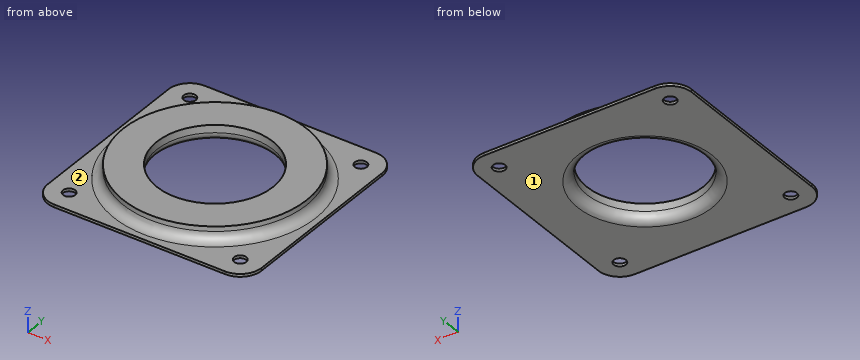
Autodesk Inventor part; units mm, degrees
ref_plane "YZ Plane" through (0, 0, 0) normal (1, 0, 0) x (0, 1, 0)
ref_plane "XZ Plane" through (0, 0, 0) normal (0, 1, 0) x (-1, 0, 0)
ref_plane "XY Plane" through (0, 0, 0) normal (0, 0, 1) x (1, 0, 0)
sketch "Skizze1" plane through (0, 0, 0) normal (0, 0, 1) x (1, 0, 0)
  line L0 (-35, 35) -> (35, 35)
  line L1 (35, 35) -> (35, -35)
  line L2 (35, -35) -> (-35, -35)
  line L3 (-35, -35) -> (-35, 35)
  circle A0 centre (0, 0) radius 35
  circle A1 centre (0, 0) radius 19
  dimension "d0" = 70
  dimension "d1" = 38
extrude "Extrusion1" add sketch "Skizze1" along normal blind 0.9
fillet "Rundung1" radius 7 4 edges at (-35, -35, 0.45) (35, -35, 0.45) (-35, 35, 0.45) (35, 35, 0.45)
sketch "Skizze2" plane through (0, 0, 0.9) normal (0, 0, 1) x (1, 0, 0)
  arc A0 (35, 28) -> (28, 35) centre (28, 28) ccw
  arc A1 (-28, 35) -> (-35, 28) centre (-28, 28) ccw
  arc A2 (-35, -28) -> (-28, -35) centre (-28, -28) ccw
  arc A3 (28, -35) -> (35, -28) centre (28, -28) ccw
  dimension "d16" = 56
hole "Bohrung1" at (-28, -28, 0.9) at (28, -28, 0.9) at (28, 28, 0.9) at (-28, 28, 0.9) direction (0, 0, -1) diameter 4 depth 8 tip angle 118
sketch "Skizze3" plane through (0, 0, 0.9) normal (0, 0, 1) x (1, 0, 0)
  circle A0 centre (0, 0) radius 19
  circle A1 centre (0, 0) radius 30
  dimension "d12" = 60
extrude "Extrusion2" add sketch "Skizze3" along normal blind 4.6
fillet "Rundung2" radius 3 2 edges at (-19, 0, 0) (-30, 0, 0.9)
properties part number "70mmkugellager" material "Stahl, galvanisiert"
Could you check a few things on this model? Use its own coordinates, in mm. Face numbers are marked on the shaded views. A direction names the side the tool comes from. Give positions to 0.01 mm unless a question says otherwise; leave off trailing zeros. Order: outer loops, then holes, each group sorted by start corner. A loop starts at its lowest first (then second) coordinate and runs counter-clockwise, first axis right, second up. Notation, with made-up numbers: (83, -25.75) - (120, -25.75) arc R28 ccw to (120, 6.25) - close; hole circle Ø9 at (-15, 11.5). An arc over 180 degrees is marked (long way). One line per question, with ' | ' between items. Start each with the question number.
Item 1: I want a section at A-A on x = 0. Write out the boundary of the cut face in (y, z).
Item 2: I'm going to push flat-ended pins straight in: pin 1 Ø2 at (x, z) = (5, 2.5) entering from -Y; pin 2 Ø8 at (x, y) = (-20.5, -12) entering from -Z; pin 3 Ø4.5 at (x, y) = (28, 28) entering from +Z. Where does each tip first touch, or does it pass through?
Item 3: I need wall thicknesses on probe 1 along Y at (x, z) = (-28, 0.65); probe 2 along Y at (x, z) = (0, 4.15). Which ranges of each line are inside material? Lowest first, please. Write a range as [from, to].
Item 4: I want a section at C-C on y = 29. Give the number of separate pieces and of enclosed holes in the cut face, then the cut area to 3 significant figures.
Item 5: For the marked faces 1 and 2, which set-ups out of +Z, -Z, +X, -X, +Y, -Y let a thin tool reach every point of the face, with its end or its side?
Verdict:
1) outline: (-35, 0) - (-22, 0) arc R3 ccw to (-19, 3) - (-19, 5.5) - (-30, 5.5) - (-30, 3.9) arc R3 cw to (-33, 0.9) - (-35, 0.9) - close; (19, 3) arc R3 ccw to (22, 0) - (35, 0) - (35, 0.9) - (33, 0.9) arc R3 cw to (30, 3.9) - (30, 5.5) - (19, 5.5) - close
2) pin 1: y = -30.81 | pin 2: z = 0 | pin 3: z = 0.9
3) probe 1: [-35, -30], [-26, 26], [30, 35] | probe 2: [-30, -19], [19, 30]
4) separate pieces: 3 | enclosed holes: 0 | area: 140 mm^2
5) face 1: -Z, +X, -X, +Y, -Y | face 2: +Z
